```python
from build123d import *

# Parameters (mm, degrees)
F1_W           = 19
F1_H           = 30
F2_DEPTH       = 75
F4_R           = 7.5
F5_DEPTH       = 5
F6_D           = 3
F6_CSINK_D     = 15
F6_CSINK_ANGLE = 90


with BuildPart() as f2:
    # F1 (on Front) → F2 (new body, symmetric)
    with BuildSketch(Plane.XZ):
        with Locations((9.5, 0)):
            Rectangle(F1_W, F1_H)
    extrude(amount=F2_DEPTH, both=True)

    # F4 (on offset) → F5 (cut, through all)
    with BuildSketch(Plane(origin=(0, 0, -10), x_dir=(1, 0, 0), z_dir=(0, 0, -1))):
        with Locations((9.5, 0)):
            Circle(F4_R)
    extrude(amount=F5_DEPTH, mode=Mode.SUBTRACT)

    # F6 (through all)
    with Locations(Plane(origin=(0, 0, -10), x_dir=(1, 0, 0), z_dir=(0, 0, -1))):
        with Locations((9.5, 0)):
            CounterSinkHole(F6_D / 2, F6_CSINK_D / 2, counter_sink_angle=F6_CSINK_ANGLE)


solid = f2.part
```
The model under review builds one solid part; all positions refer to its coordinate system, in mm. A direction names the side the tool comes from. Coordinates: 2 decimals unless noted, no trailing zeros. Write each loop counter-clockwise with the first axis right and the second up, starting at its lowest first coordinate (ties: lowest second). Pieces come first, ordered by that corner, then holes. Notation, with made-up numbers: (0, 6) - (21, 6) arc R34 ccw to (21, 43) - close; hole circle Ø2 at (-16, -27.5). An arc over 180 degrees is marked (long way). Answer in a Markdown table with one row per item. Add a question column.
Q1. To check wall thickness, follow line 1 along X through (y, z) = (0, -12.35); line 2 along Y through (x, z) = (9.5, -12.95); line 3 along Y through (x, z) = (9.5, 5). State the ranges of each line that lie inside material, in increasing order. Write a range as from..to.
Q2. Consider section A-A on y = 0. Give the boundary of the cut face in (x, z).
Q3. Draft analysis for pull direction X (two halves, no side actions). For faces 1 (the face through (19, -1, 0)), 2 (the face through (11, 0, 6)), 3 (the face through (9, 75, 0)), state which applies: +X half, -X half, draft (parallel to the pull), parting line (faces both ways), or undercut.
Q4. Clearance check with flat-ended pins moving along their axes: pin 1 (9 mm diameter, centred on x = 9.5, y = 0, fed in from -Z); pin 2 (2.5 mm diameter, centred on x = 9.5, y = 0, fed in from +Z). State where each tip first meets the part, or that it passes through.
Q5. Consider section B-B on x = 9.5. Give the boundary of the cut face in (y, z), then the cut area to 3 significant figures.
Q6. For faces 4 (the face through (2, 0, -12)), 5 (the face through (7, -1, 15)), list the 3-axis set-ups (+Z, -Z, +X, -X, +Y, -Y) from which the entire face can be reached by the end or side of a thin tool; tool diameter is ignored.
Answers below:
| question | item | result |
|---|---|---|
| 1 | line 1 | 0..2, 17..19 |
| 1 | line 2 | -75..-7.5, 7.5..75 |
| 1 | line 3 | -75..-1.5, 1.5..75 |
| 2 | outline | (0, -15) - (2, -15) - (2, -10) - (8, -4) - (8, 15) - (0, 15) - close; (11, -4) - (17, -10) - (17, -15) - (19, -15) - (19, 15) - (11, 15) - close |
| 3 | face 1 | +X half |
| 3 | face 2 | undercut |
| 3 | face 3 | draft |
| 4 | pin 1 | z = -7 |
| 4 | pin 2 | through |
| 5 | outline | (-75, -15) - (-7.5, -15) - (-7.5, -10) - (-1.5, -4) - (-1.5, 15) - (-75, 15) - close; (1.5, -4) - (7.5, -10) - (7.5, -15) - (75, -15) - (75, 15) - (1.5, 15) - close |
| 5 | area | 4,310 mm² |
| 6 | face 4 | -Z |
| 6 | face 5 | +Z, +X, -X, +Y, -Y |
